The figure shows three views and two pictorial views of one solid part (mm, origin at its lowest corner). Answer the questions. A direction names the side the tool comes from. Give positions to 0.01 mm unless a question says otherwise; leave off trailing zeros. Loops run counter-clockwise (first coordinate to the right, second up) from the corner with the lowest first, then second, coordinate; pieces in that order, holes last. Notation, with made-up numbers: M 25.5,-21.75 L 83.5,-21.75 A12 ccw 83.5,-0.75 Z; hole C 36,24 d1. An arc over 180 degrees is marked long. One line per item, written item: value. Start each with the question number.
Q1. The mould has two halves that part along Z. Classify the marked faces 6, 7, 8 and 9: +Z half, -Z half, draft (parallel to the pull), parting line (faces both ways), or undercut.
Q2. Flat-ended cylindrical pins translate along their axes: pin 1 (4.5 mm diameter, centred on x = 6.35, y = 139.84, fed in from -Z); pin 2 (4 mm diameter, centred on x = 7, z = 10, fed in from -Y); pin 3 (4 mm diameter, centred on y = 160, z = 83.5, fed in from +X); pin 4 (10 mm diameter, centred on y = 54.5, z = 70, fed in from -X) (1 decimal). Find the tip coordinate at first contact, or state that the pin passes through.
Q3. A cutting plane is placed at C-C, the plane z = 60. Determine the outline of the cut face in (x, y).
Q4. Consider L1, parallel to Z at x = 19, y = 9; L2, parallel to Z at x = 5, y = 77; L3, parallel to Y at x = 6, z = 79 (1 decimal). Determine where each line is inside the solid, lowest interval first.
Q5. For the marked faces 1, 2, 3, 4 and 5, determine the directions among +Z, -Z, +X, -X, +Y, -Y from which every point of the face is accessible in a straight line to the end or side of a thin tool.
Q6. A cutting plane is placed at D-D, the plane z = 22.5. Determine the outline of the cut face in (x, y).
Q7. A cutting plane is placed at B-B, the plane z = 83. State how many separate pieces and enclosed holes the cut face has, and give its area (3 significant figures).
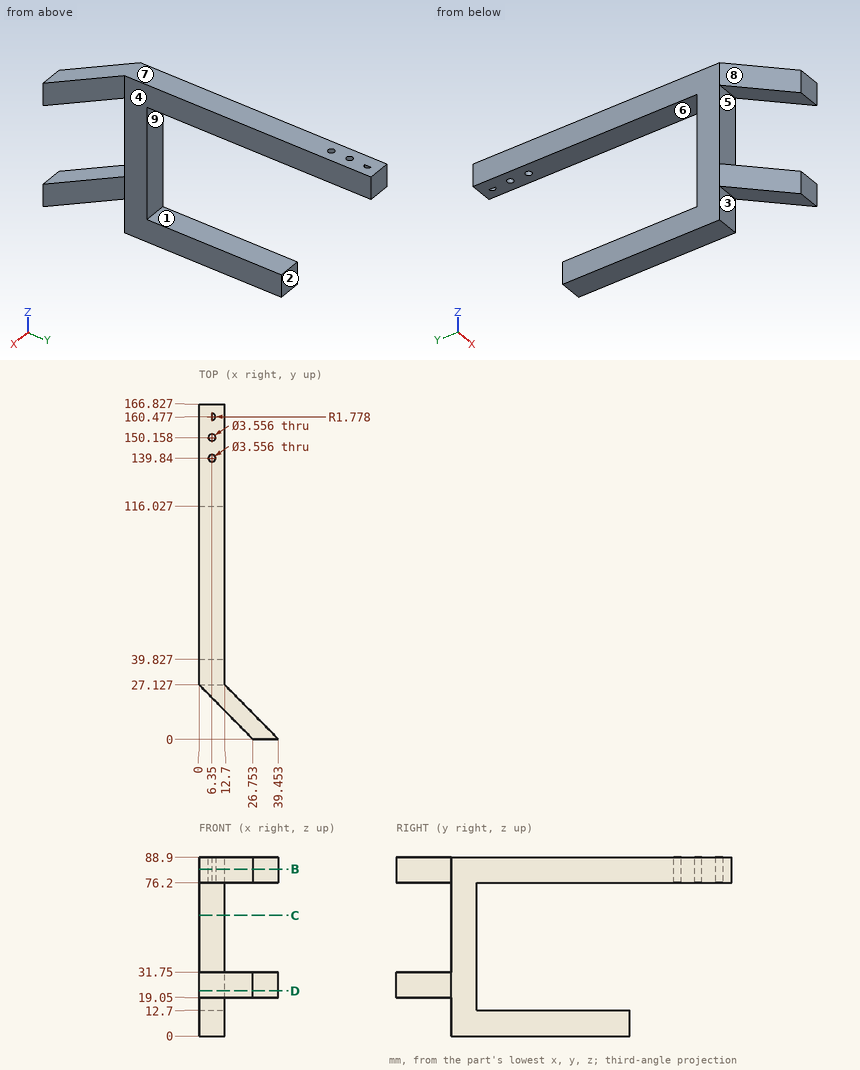
Answer block:
1. face 6: undercut
1. face 7: +Z half
1. face 8: draft
1. face 9: undercut
2. pin 1: z = 76.2
2. pin 2: y = 27.13
2. pin 3: x = 12.7
2. pin 4: through
3. outline: M 0,27.13 L 12.7,27.13 L 12.7,39.83 L 0,39.83 Z
4. L1: 19.05 to 31.75, 76.2 to 88.9
4. L2: 0 to 12.7, 76.2 to 88.9
4. L3: 21 to 138.1, 141.6 to 148.4, 151.9 to 166.8
5. face 1: +X, -X, +Y
5. face 2: -Z, +X, -X, +Y
5. face 3: -Z, +X, -X, -Y
5. face 4: +Z, -Z, +X, +Y
5. face 5: +X, -X, -Y
6. outline: M 0,27.13 L 26.75,0 L 39.45,0 L 12.7,27.13 L 12.7,39.83 L 0,39.83 Z
7. separate pieces: 1
7. enclosed holes: 3
7. area: 2,090 mm^2
